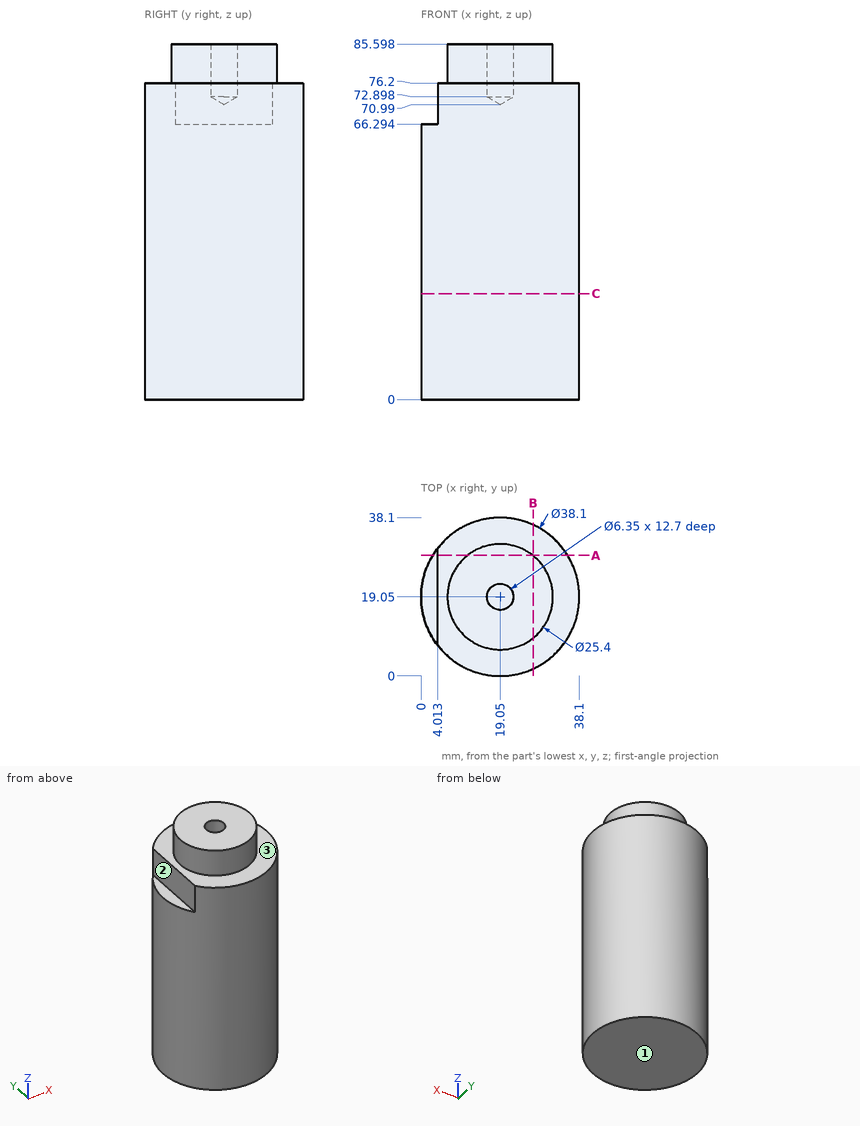
Design review of the part shown in the three views and the two pictorial views. Dimensions are in mm from the part's minimum x, y and z. A direction names the side the tool comes from. Round coordinates to 2 decimals unless told otherwise and drop trailing zeros. Write each loop counter-clockwise with the first axis right and the second up, starting at its lowest first coordinate (ties: lowest second). Pieces come first, ordered by that corner, then holes. Notation, with made-up numbers: (26, -24.5) - (81, -24.5) arc R23 ccw to (81, 9.5) - close; hole circle Ø6 at (66, 37.5). An arc over 180 degrees is marked (long way). Write item = value, one per line. Start each with the question number.
1. For pin 1 Ø8 at (x, z) = (27, 57.5) entering from -Y; pin 2 Ø10 at (x, z) = (30.5, 15.5) entering from +Y (1 decimal); pin 3 Ø2 at (x, y) = (1, 20) entering from +Z, all flat-tipped, find the tip position at first contact; note any pin that passes through.
2. For the marked faces 1, 2 and 3, list the 3-axis set-ups (+Z, -Z, +X, -X, +Y, -Y) from which the entire face can be reached by the end or side of a thin tool; tool diameter is ignored.
3. Consider section A-A on y = 29. State the section outline as (x, z) points (1 decimal).
4. Consider section C-C on z = 25.5. State the section outline as (x, y) points, plus the area to 3 significant figures.
5. Wall thickness on L1, parallel to Z at x = 3, y = 10.5; L2, parallel to Z at x = 24, y = 35; L3, parallel to X at y = 13, z = 76.5: over which ranges is each line inside the solid? List them lowest first.
6. Consider section B-B on x = 27. State the section outline as (y, z) points, plus the area to 3 significant figures.
Evaluation:
q1.pin_1 = 0.41
q1.pin_2 = 37
q1.pin_3 = 66.29
q2.face_1 = -Z, +X, -X, +Y, -Y
q2.face_2 = +Z, -X, +Y, -Y
q2.face_3 = +Z
q3.outline = (2.8, 0) - (35.3, 0) - (35.3, 76.2) - (26.9, 76.2) - (26.9, 85.6) - (11.2, 85.6) - (11.2, 76.2) - (4, 76.2) - (4, 66.3) - (2.8, 66.3) - close
q4.outline = circle Ø38.1 at (19.05, 19.05)
q4.area = 1,140 mm2
q5.L1 = 0 to 66.29
q5.L2 = 0 to 76.2
q5.L3 = 7.88 to 30.22
q6.outline = (1.74, 0) - (36.36, 0) - (36.36, 76.2) - (28.95, 76.2) - (28.95, 85.6) - (9.15, 85.6) - (9.15, 76.2) - (1.74, 76.2) - close
q6.area = 2,820 mm2
